Input: part model. Units: mm. Frame: model coordinates. A direction names the side the tool comes from. Coordinates: 2 decimals unless noted, no trailing zeros. Loops run counter-clockwise (first coordinate to the right, second up) from the corner with the lowest first, then second, coordinate; pieces in that order, holes last. Notation, with made-up numbers: (66, -18.5) - (79, -18.5) arc R24 cw to (79, 11.5) - close; hole circle Ø10 at (56, 62.5). An arc over 180 degrees is marked (long way). Write item = value, one per line. Start each with the question number.
Autodesk Inventor part; units mm, degrees
ref_plane "YZ Plane" through (0, 0, 0) normal (1, 0, 0) x (0, 1, 0)
ref_plane "XZ Plane" through (0, 0, 0) normal (0, 1, 0) x (-1, 0, 0)
ref_plane "XY Plane" through (0, 0, 0) normal (0, 0, 1) x (1, 0, 0)
sketch "Sketch1" plane through (0, 0, 0) normal (0, 0, 1) x (1, 0, 0)
  line L0 (0, 0) -> (50, 0)
  line L1 (50, 0) -> (50, 15)
  line L2 (50, 15) -> (0, 15)
  line L3 (0, 15) -> (0, 0)
  circle A0 centre (5.95, 6.5) radius 1.5
  circle A1 centre (44.05, 6.5) radius 1.5
  dimension "d0" = 50
  dimension "d1" = 15
  dimension "d4" = 3
  dimension "d5" = 3
  dimension "d6" = 38.1
  dimension "d7" = 5.95
  dimension "d8" = 6.5
  dimension "d9" = 6.5
extrude "Extrusion1" add sketch "Sketch1" along normal blind 1.7
sketch "Sketch2" plane through (0, 0, 1.7) normal (0, 0, 1) x (1, 0, 0)
  line L0 (9.03, 2.67) -> (40.43, 2.67)
  line L1 (40.43, 2.67) -> (40.43, 0.17)
  line L2 (40.43, 0.17) -> (9.03, 0.17)
  line L3 (9.03, 0.17) -> (9.03, 2.67)
  circle A0 centre (5.95, 6.5) radius 1.5
  point P0 (0, 0)
  dimension "d10" = 31.4
  dimension "d11" = 2.5
  dimension "d12" = 3.83
  dimension "d13" = 3.08
extrude "Extrusion2" add sketch "Sketch2" along normal blind 10 contours L0 L1 L2 L3
properties part number "DeviceConnector"
Item 1: Cut plane D-D on x = 18. Return loops of the section in (y, z).
Item 2: Access query for faces 1 (the flat face through (25, 2.67, 7)), 2 (the flat face through (40.43, 1, 7)), 3 (the flat face through (50, 7, 1)), 4 (the flat face through (25, 0.17, 7)). Directions: +Z, -Z, +X, -X, +Y, -Y. A direction counts if a zero-diameter tool reaches every point of the face in a straight line with its end or side. Return the directions, or none.
Item 3: Ray query, line 1 (Y direction, x = 5.95, z = 0.6); line 2 (Z direction, x = 36.5, y = 6); line 3 (Y direction, x = 27, z = 2). Return the intervals inside material, ascending.
Item 4: Cut plane C-C on y = 1.75. Return loops of the section in (x, z).
Item 5: Pull-direction query (X, two-part tool) for faces 5 (the flat face through (9.03, 1, 7)), 6 (the cylindrical face through (45.48, 6.05, 0.84)), 7 (the flat face through (25, 0, 1)); classes: pulls with the +X half, pulls with the -X half, needs draft (parallel to the pull), parting line crosses it, or undercut.
Item 6: Cut plane A-A on y = 6.5. Return loops of the section in (x, z), plus the area to 3 significant figures.
Item 7: Pin query (flat end, axial travel): pin 1 (1.5 mm diameter, centred on y = 2.5, z = 4.5, fed in from -X); pin 2 (6 mm diameter, centred on x = 20.5, z = 7.5, fed in from -Y); pin 3 (1.2 mm diameter, centred on y = 1.5, z = 7.5, fed in from +X). Return the tip coordinate at first contact, or that it passes through.
Item 8: Cut plane B-B on x = 44.05. Return loops of the section in (y, z).
Recorded:
q1.outline = (0, 0) - (15, 0) - (15, 1.7) - (2.67, 1.7) - (2.67, 11.7) - (0.17, 11.7) - (0.17, 1.7) - (0, 1.7) - close
q2.face_1 = +Z, +X, -X, +Y
q2.face_2 = +Z, +X, +Y, -Y
q2.face_3 = +Z, -Z, +X, +Y, -Y
q2.face_4 = +Z, +X, -X, -Y
q3.line_1 = 0 to 5, 8 to 15
q3.line_2 = 0 to 1.7
q3.line_3 = 0.17 to 2.67
q4.outline = (0, 0) - (50, 0) - (50, 1.7) - (40.43, 1.7) - (40.43, 11.7) - (9.03, 11.7) - (9.03, 1.7) - (0, 1.7) - close
q5.face_5 = pulls with the -X half
q5.face_6 = undercut
q5.face_7 = needs draft
q6.outline = (0, 0) - (4.45, 0) - (4.45, 1.7) - (0, 1.7) - close; (7.45, 0) - (42.55, 0) - (42.55, 1.7) - (7.45, 1.7) - close; (45.55, 0) - (50, 0) - (50, 1.7) - (45.55, 1.7) - close
q6.area = 74.8 mm²
q7.pin_1 = 9.03
q7.pin_2 = 0.17
q7.pin_3 = 40.43
q8.outline = (0, 0) - (5, 0) - (5, 1.7) - (0, 1.7) - close; (8, 0) - (15, 0) - (15, 1.7) - (8, 1.7) - close
